Check sheet for the modelled part. Datum: model origin and axes. Units: mm. A direction names the side the tool comes from. Round coordinates to 2 decimals unless told otherwise and drop trailing zeros. One line per item, written item: value.
from build123d import *

# Parameters (mm, degrees)
F1_DEPTH = 10


with BuildPart() as f1:
    # F0 (on Top) → F1 (new body)
    with BuildSketch(Plane.XY):
        with BuildLine():
            Line((40, 5), (-40, 5))
            Line((-40, 5), (-40, -5))
            Line((-40, -5), (-1.496606, -5))
            Line((-1.496606, -5), (-0.92388, -3.617317))
            ThreePointArc((-0.92388, -3.617317), (0, -3), (0.92388, -3.617317))
            Line((0.92388, -3.617317), (1.496606, -5))
            Line((1.496606, -5), (40, -5))
            Line((40, -5), (40, 5))
        make_face()
    extrude(amount=F1_DEPTH)


solid = f1.part
Q1. Scan lines: line 1 (X direction, y = -4, z = 2); line 2 (X direction, y = -3.5, z = 6.75); line 3 (Y direction, x = 0.5, z = 4). Record each from-to range of solid material in increasing order. Write a range as [from, to].
Completed:
line 1: [-40, -1.08], [1.08, 40]
line 2: [-40, -0.87], [0.87, 40]
line 3: [-3.13, 5]
Q2. Access from +Z, -Z, +X, -X, +Y, -Y to the whole of each face (thin tool, end or side, straight path). Record for faces 4 (the flat face through (-1.214, -4.318, 4.93)), 5 (the flat face through (20, -5, 5)).
Completed:
face 4: +Z, -Z, -Y
face 5: +Z, -Z, +X, -X, -Y
Q3. Draft check along X on faces 1 (the flat face through (-40, 0, 5)), 2 (the cylindrical face through (0, -3, 5)), 3 (the flat face through (1, 5, 5)). Enter one of: pulls with the +X half, pulls with the -X half, needs draft (parallel to the pull), parting line crosses it, or undercut.
Completed:
face 1: pulls with the -X half
face 2: undercut
face 3: needs draft
